from build123d import *

# Parameters (mm, degrees)
BOSS_EXTRUDE1_DEPTH     = 17
SKETCH2_R               = 10.5
BOSS_EXTRUDE2_DEPTH     = 58
SKETCH3_R               = 12.5
BOSS_EXTRUDE3_DEPTH     = 13.5
SKETCH4_R               = 7.55
SKETCH4_R_2             = 5.15
CUT_EXTRUDE1_DEPTH      = 59
SKETCH5_R               = 4.05
CUT_EXTRUDE2_DEPTH      = 35
SKETCH6_R               = 2.293291756
SKETCH6_R_2             = 2.82251293
SKETCH6_R_3             = 2.373314239
CUT_EXTRUDE3_DEPTH      = 18
CUT_EXTRUDE4_DEPTH      = 20
SKETCH10_R              = 1.875
CUT_EXTRUDE6_DEPTH      = 59
SKETCH11_W              = 1
SKETCH11_H              = 2
CUT_EXTRUDE7_DEPTH      = 8
CUT_EXTRUDE9_DEPTH      = 1
CUT_EXTRUDE9_DEPTH_BACK = 57


with BuildPart() as part:
    # Sketch1 → Boss-Extrude1 (new body)
    with BuildSketch(Plane.XY):
        with BuildLine():
            Line((39, -53), (48, -53))
            Line((48, -53), (51.5, -49.5))
            Line((51.5, -49.5), (51.5, -44))
            Line((51.5, -44), (44.75, -32.029420251))
            ThreePointArc((44.75, -32.029420251), (44.267998826, -30.444746543), (44.500869457, -28.804841922))
            Line((44.500869457, -28.804841922), (45.840453499, -25.237554933))
            ThreePointArc((45.840453499, -25.237554933), (51.941858088, -17.410271227), (61.414466094, -14.45))
            Line((61.414466094, -14.45), (63.414466094, -14.45))
            ThreePointArc((63.414466094, -14.45), (66.680873506, -15.099728831), (69.45, -16.95))
            Line((69.45, -16.95), (72.95, -20.45))
            Line((72.95, -20.45), (77.45, -20.45))
            Line((77.45, -20.45), (79.45, -18.45))
            Line((79.45, -18.45), (79.45, -4.45))
            Line((79.45, -4.45), (75, 0))
            Line((75, 0), (39, 0))
            Line((39, 0), (0, 0))
            Line((0, 0), (0, -58))
            Line((0, -58), (39, -58))
            Line((39, -58), (39, -53))
        make_face()
    extrude(amount=BOSS_EXTRUDE1_DEPTH)

    # Sketch2 → Boss-Extrude2 (add)
    with BuildSketch(Plane(origin=(0, 0, 0), x_dir=(1, 0, 0), z_dir=(0, 1, 0))):
        with Locations((26.427, 6.5)):
            Circle(SKETCH2_R)
    extrude(amount=-BOSS_EXTRUDE2_DEPTH)

    # Sketch3 → Boss-Extrude3 (add)
    with BuildSketch(Plane(origin=(0, 0, 0), x_dir=(1, 0, 0), z_dir=(0, 1, 0))):
        with Locations((10.677078252, 6.5)):
            Circle(SKETCH3_R)
    extrude(amount=-BOSS_EXTRUDE3_DEPTH)

    # Sketch4 → Cut-Extrude1 (cut, through all)
    with BuildSketch(Plane(origin=(0, 0, 0), x_dir=(1, 0, 0), z_dir=(0, 1, 0))):
        with Locations((26.427, 6.5)):
            Circle(SKETCH4_R)
        with Locations((10.677078252, 6.5)):
            Circle(SKETCH4_R_2)
    extrude(amount=-CUT_EXTRUDE1_DEPTH, mode=Mode.SUBTRACT)

    # Sketch5 → Cut-Extrude2 (cut)
    with BuildSketch(Plane.ZY):
        with Locations((8.5, -6)):
            Circle(SKETCH5_R)
        with Locations((8.5, -51)):
            Circle(SKETCH5_R)
        Polygon((10.5, -43.5), (6.65, -43.5), (3.65, -38), (3.65, -19), (6.65, -13.5), (10.5, -13.5), (13.5, -19), (13.5, -38), align=None)
    extrude(amount=-CUT_EXTRUDE2_DEPTH, mode=Mode.SUBTRACT)

    # Sketch6 → Cut-Extrude3 (cut, through all)
    with BuildSketch(Plane(origin=(0, 0, 0), x_dir=(-1, 0, 0), z_dir=(0, 0, -1))):
        with Locations((-75.950256659, -13)):
            Circle(SKETCH6_R)
        with Locations((-44.950256659, -13)):
            Circle(SKETCH6_R_2)
        with Locations((-44.950256659, -44)):
            Circle(SKETCH6_R_3)
    extrude(amount=-CUT_EXTRUDE3_DEPTH, mode=Mode.SUBTRACT)

    # Sketch8 → Cut-Extrude4 (cut)
    with BuildSketch(Plane.ZY.offset(-35)):
        Polygon((10.5, -43.5), (13.5, -38), (13.5, -19), (10.5, -13.5), (6.65, -13.5), (3.65, -19), (3.65, -38), (6.65, -43.5), align=None)
    extrude(amount=-CUT_EXTRUDE4_DEPTH, mode=Mode.SUBTRACT)

    # Sketch10 → Cut-Extrude6 (cut, through all)
    with BuildSketch(Plane(origin=(0, 0, 0), x_dir=(1, 0, 0), z_dir=(0, 1, 0))):
        with Locations((13.570159095, 14.092477082)):
            Circle(SKETCH10_R)
        with Locations((3.08460117, 9.393080843)):
            Circle(SKETCH10_R)
    extrude(amount=-CUT_EXTRUDE6_DEPTH, mode=Mode.SUBTRACT)

    # Sketch11 → Cut-Extrude7 (cut)
    with BuildSketch(Plane.XZ.offset(58)):
        with Locations((34.5, 9.5)):
            Rectangle(SKETCH11_W, SKETCH11_H)
    cut_extrude7 = extrude(amount=-CUT_EXTRUDE7_DEPTH, mode=Mode.SUBTRACT)

    # Mirror1: Cut-Extrude7 across plane
    add(cut_extrude7.mirror(Plane.ZX.offset(-29)), mode=Mode.SUBTRACT)

    # Sketch13 → Cut-Extrude9 (cut, two sides)
    with BuildSketch(Plane.XZ.offset(58)) as cut_extrude9_sk:
        with BuildLine():
            Line((147.448117004, -6.5), (36.927, -6.5))
            Line((36.927, -6.5), (33.977, -6.5))
            ThreePointArc((33.977, -6.5), (33.912408703, -7.485472751), (33.719739988, -8.454083791))
            Line((33.719739988, -8.454083791), (36.569221176, -9.217599974))
            Line((36.569221176, -9.217599974), (143.32442244, -37.82256994))
            Line((143.32442244, -37.82256994), (362.475609494, -66.674371065))
            Line((362.475609494, -66.674371065), (366.599304057, -35.351801125))
            Line((366.599304057, -35.351801125), (147.448117004, -6.5))
        make_face()
    extrude(amount=CUT_EXTRUDE9_DEPTH, mode=Mode.SUBTRACT)
    extrude(cut_extrude9_sk.sketch, amount=-CUT_EXTRUDE9_DEPTH_BACK, mode=Mode.SUBTRACT)


solid = part.part
Model file for the job. Use its own axes, mm. A direction names the side the tool comes from. Give positions to 0.01 mm unless a question says otherwise; leave off trailing zeros. Write each loop counter-clockwise with the first axis right and the second up, starting at its lowest first coordinate (ties: lowest second). Pieces come first, ordered by that corner, then holes. Notation, with made-up numbers: M -22.75,16.25 L -10.75,16.25 A26 ccw -10.75,54.25 Z; hole C -11,-2 d11. An arc over 180 degrees is marked long. One line per item, written item: value. Start each with the question number.
Q1. Two-plate mould, pull along Z, no slides. Class faces 5 (the flat face through (49.672, -40.759, 4.603)), 6 (the cylindrical face through (13.05, -6.66, -1.93)): +Z half, -Z half, draft (parallel to the pull), parting line (faces both ways), or undercut.
Q2. Probe probe 1 along Z at (x, y) = (2, -25.5); probe 2 along X at (y, z) = (-4.5, -11); probe 3 along Y at (x, z) = (17, 8). List the from-to ranges inside material, lowest first. Write a range as [from, to].
Q3. 3-axis set-ups, long thin cutter, end or side, ignore diameter. For faces 1 (the cylindrical face through (17.255, -8.464, 5.286)), 2 (the flat face through (43, -53, 8)), 3 (the cylindrical face through (66.637, -15.082, 8.381)), 4 (the flat face through (49, -43.5, 9)): which of +Z, -Z, +X, -X, +Y, -Y reach the whole face in a straight line?
Q4. Saw through at C-C, the plane z = -3. Write the cut outline in (x, y), plus the area to 3 significant figures.
Q5. Saw through at D-D, the plane y = -51. Write the cut outline in (x, z), plus the area to 3 significant figures.
Q6. Drop flat-ended pins along their axis: pin 1 Ø9.5 at (y, z) = (-51, 8.5) entering from +X; pin 2 Ø1.5 at (y, z) = (-49, -4) entering from -X; pin 3 Ø3.5 at (x, y) = (75.95, -13) entering from +Z; pin 4 Ø5 at (x, z) = (74, 11.5) entering from -Y. Give the stop position or say it passes through.
Q7. Saw through at A-A, the plane x = 8.5. Write the cut outline in (y, z), plus the area to 3 significant figures.
Q8. Saw through at B-B, the plane y = -39.5. Write the cut outline in (x, z).
Output values:
1. face 5: draft
1. face 6: undercut
2. probe 1: z = [0, 3.65], [13.5, 17]
2. probe 2: x = [-0.98, 2.12], [4.05, 8.17], [13.18, 20.36], [32.49, 35.91]
2. probe 3: y = [-58, -55.02], [-46.98, -43.5], [-13.5, -10.02], [-1.98, 0]
3. face 1: -X
3. face 2: +Z, -Z, +X, -Y
3. face 3: +Z, -Z, -Y
3. face 4: +X, -X
4. outline: M -1.32,-13.5 L 6.9,-13.5 L 6.9,0 L -1.32,0 Z; M 14.45,-13.5 L 16.53,-13.5 L 16.53,-58 L 19.74,-58 L 19.74,0 L 14.45,0 Z; M 33.12,-58 L 36.33,-58 L 36.33,0 L 33.12,0 Z
4. area: 511 mm²
5. outline: M 0,0 L 18.18,0 A10.5 ccw long 36.57,-9.22 L 33.72,-8.45 A7.55 cw long 33.98,-6.5 L 36.93,-6.5 A10.5 ccw 34.67,0 L 50,0 L 50,17 L 0,17 L 0,12.55 L 35,12.55 L 35,4.45 L 0,4.45 Z
5. area: 681 mm²
6. pin 1: stops at x = 51.5
6. pin 2: stops at x = 16.07
6. pin 3: passes through
6. pin 4: stops at y = -20.45
7. outline: M -58,0 L -13.5,0 L -13.5,-1.83 L 0,-1.83 L 0,17 L -58,17 Z; M -13.5,-18.81 L 0,-18.81 L 0,-11.17 L -13.5,-11.17 Z; hole C -51,8.5 d8.1; hole M -43.5,6.65 L -38,3.65 L -19,3.65 L -13.5,6.65 L -13.5,10.5 L -19,13.5 L -38,13.5 L -43.5,10.5 Z; hole C -6,8.5 d8.1
7. area: 748 mm²
8. outline: M 0,0 L 18.18,0 A10.5 ccw long 36.57,-9.22 L 33.72,-8.45 A7.55 cw long 33.98,-6.5 L 36.93,-6.5 A10.5 ccw 34.67,0 L 48.96,0 L 48.96,4.47 L 0,4.47 Z; M 0,12.68 L 48.96,12.68 L 48.96,17 L 0,17 Z
